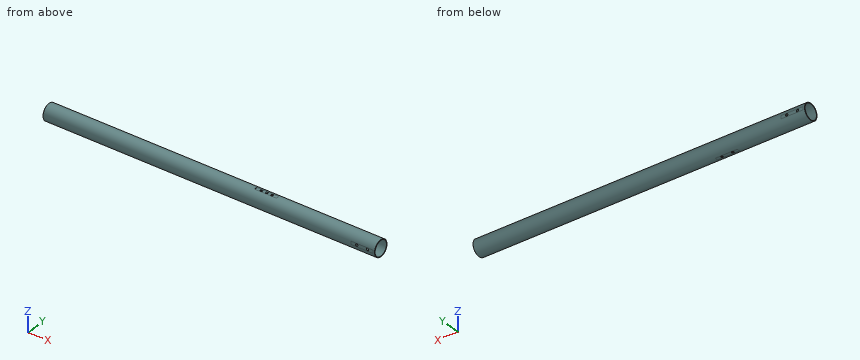
from build123d import *

# Parameters (mm, degrees)
SKETCH1_R                     = 25
SKETCH1_R_2                   = 23
EXTRUDE_THIN1_DEPTH           = 515
EXTRUDE_THIN2_START           = 210
SKETCH1_3_R                   = 25
SKETCH1_3_R_2                 = 21
EXTRUDE_THIN2_DEPTH           = 90
CUT_EXTRUDE1_START            = 24.54
CUT_EXTRUDE1_DEPTH            = 492.672165684
CUT_EXTRUDE2_START            = -24.54
CUT_EXTRUDE2_DEPTH            = 492.672165793
CUT_EXTRUDE3_START            = -24.54
CUT_EXTRUDE3_DEPTH            = 492.672165793
CUT_EXTRUDE4_START            = 24.54
CUT_EXTRUDE4_DEPTH            = 492.672165793
M_0_295_DIAMETER_HOLE3_REACH  = 519.981
M_0_295_DIAMETER_HOLE3_BORE_R = 3.7465
M_0_295_DIAMETER_HOLE4_REACH  = 519.981
M_0_295_DIAMETER_HOLE4_BORE_R = 3.7465
M_0_295_DIAMETER_HOLE5_REACH  = 519.981
M_0_295_DIAMETER_HOLE5_BORE_R = 3.7465
M_0_295_DIAMETER_HOLE6_REACH  = 519.981
M_0_295_DIAMETER_HOLE6_BORE_R = 3.7465
CHAMFER1_SIZE                 = 1


with BuildPart() as part:
    # Sketch1 → Extrude-Thin1 (new, symmetric)
    with BuildSketch(Plane(origin=(0, 0, 0), x_dir=(0, 0, -1), z_dir=(1, 0, 0))):
        Circle(SKETCH1_R)
        Circle(SKETCH1_R_2, mode=Mode.SUBTRACT)
    extrude(amount=EXTRUDE_THIN1_DEPTH, both=True)

    # Sketch1<3> → Extrude-Thin2 (add)
    with BuildSketch(Plane(origin=(0, 0, 0), x_dir=(0, 0, -1), z_dir=(1, 0, 0)).offset(EXTRUDE_THIN2_START)):
        Circle(SKETCH1_3_R)
        Circle(SKETCH1_3_R_2, mode=Mode.SUBTRACT)
    extrude(amount=-EXTRUDE_THIN2_DEPTH)

    # Sketch3 → Cut-Extrude1 (cut, through all)
    with BuildSketch(Plane(origin=(0, 0, 0), x_dir=(1, 0, 0), z_dir=(0, 1, 0)).offset(CUT_EXTRUDE1_START)):
        with BuildLine():
            Line((-491.7775, -17.4725), (-458.1225, -17.4725))
            ThreePointArc((-458.1225, -17.4725), (-440.65, 0), (-458.1225, 17.4725))
            Line((-458.1225, 17.4725), (-491.7775, 17.4725))
            ThreePointArc((-491.7775, 17.4725), (-509.25, 0), (-491.7775, -17.4725))
        make_face()
    extrude(amount=CUT_EXTRUDE1_DEPTH, mode=Mode.SUBTRACT)

    # Sketch8 → Cut-Extrude2 (cut, through all)
    with BuildSketch(Plane.XY.offset(CUT_EXTRUDE2_START)):
        with BuildLine():
            Line((-272.5275, -17.4725), (-238.8725, -17.4725))
            ThreePointArc((-238.8725, -17.4725), (-221.4, 0), (-238.8725, 17.4725))
            Line((-238.8725, 17.4725), (-272.5275, 17.4725))
            ThreePointArc((-272.5275, 17.4725), (-290, 0), (-272.5275, -17.4725))
        make_face()
    extrude(amount=-CUT_EXTRUDE2_DEPTH, mode=Mode.SUBTRACT)

    # Sketch3<3> → Cut-Extrude3 (cut, through all)
    with BuildSketch(Plane(origin=(0, 0, 0), x_dir=(1, 0, 0), z_dir=(0, 1, 0)).offset(CUT_EXTRUDE3_START)):
        with BuildLine():
            ThreePointArc((458.1225, -17.4725), (440.65, 0), (458.1225, 17.4725))
            Line((458.1225, 17.4725), (491.7775, 17.4725))
            ThreePointArc((491.7775, 17.4725), (509.25, 0), (491.7775, -17.4725))
            Line((491.7775, -17.4725), (458.1225, -17.4725))
        make_face()
    extrude(amount=-CUT_EXTRUDE3_DEPTH, mode=Mode.SUBTRACT)

    # Sketch8<4> → Cut-Extrude4 (cut, through all)
    with BuildSketch(Plane.XY.offset(CUT_EXTRUDE4_START)):
        with BuildLine():
            Line((143.8725, -17.4725), (177.5275, -17.4725))
            ThreePointArc((177.5275, -17.4725), (195, 0), (177.5275, 17.4725))
            Line((177.5275, 17.4725), (143.8725, 17.4725))
            ThreePointArc((143.8725, 17.4725), (126.4, 0), (143.8725, -17.4725))
        make_face()
    extrude(amount=CUT_EXTRUDE4_DEPTH, mode=Mode.SUBTRACT)

    # M (0.295) Diameter Hole3 bore → M (0.295) Diameter Hole3 (cut, up to next)
    with BuildSketch(Plane(origin=(0, 24.54, 0), x_dir=(1, 0, 0), z_dir=(0, 1, 0)), mode=Mode.PRIVATE) as m_0_295_diameter_hole3_sk1:
        with Locations((-491.7775, 0)):
            Circle(M_0_295_DIAMETER_HOLE3_BORE_R)
    m_0_295_diameter_hole3_tool1 = extrude(m_0_295_diameter_hole3_sk1.sketch, amount=-M_0_295_DIAMETER_HOLE3_REACH, mode=Mode.PRIVATE) & part.part
    # M (0.295) Diameter Hole3 bore → M (0.295) Diameter Hole3 (cut, up to next)
    with BuildSketch(Plane(origin=(0, 24.54, 0), x_dir=(1, 0, 0), z_dir=(0, 1, 0)), mode=Mode.PRIVATE) as m_0_295_diameter_hole3_sk2:
        with Locations((-458.1225, 0)):
            Circle(M_0_295_DIAMETER_HOLE3_BORE_R)
    m_0_295_diameter_hole3_tool2 = extrude(m_0_295_diameter_hole3_sk2.sketch, amount=-M_0_295_DIAMETER_HOLE3_REACH, mode=Mode.PRIVATE) & part.part
    add(m_0_295_diameter_hole3_tool1.solids().sort_by_distance((-491.7775, 24.54, 0))[0], mode=Mode.SUBTRACT)
    add(m_0_295_diameter_hole3_tool2.solids().sort_by_distance((-458.1225, 24.54, 0))[0], mode=Mode.SUBTRACT)

    # M (0.295) Diameter Hole4 bore → M (0.295) Diameter Hole4 (cut, up to next)
    with BuildSketch(Plane(origin=(0, 0, -24.54), x_dir=(-1, 0, 0), z_dir=(0, 0, -1)), mode=Mode.PRIVATE) as m_0_295_diameter_hole4_sk1:
        with Locations((238.8725, 0)):
            Circle(M_0_295_DIAMETER_HOLE4_BORE_R)
    m_0_295_diameter_hole4_tool1 = extrude(m_0_295_diameter_hole4_sk1.sketch, amount=-M_0_295_DIAMETER_HOLE4_REACH, mode=Mode.PRIVATE) & part.part
    # M (0.295) Diameter Hole4 bore → M (0.295) Diameter Hole4 (cut, up to next)
    with BuildSketch(Plane(origin=(0, 0, -24.54), x_dir=(-1, 0, 0), z_dir=(0, 0, -1)), mode=Mode.PRIVATE) as m_0_295_diameter_hole4_sk2:
        with Locations((272.5275, 0)):
            Circle(M_0_295_DIAMETER_HOLE4_BORE_R)
    m_0_295_diameter_hole4_tool2 = extrude(m_0_295_diameter_hole4_sk2.sketch, amount=-M_0_295_DIAMETER_HOLE4_REACH, mode=Mode.PRIVATE) & part.part
    add(m_0_295_diameter_hole4_tool1.solids().sort_by_distance((-238.8725, 0, -24.54))[0], mode=Mode.SUBTRACT)
    add(m_0_295_diameter_hole4_tool2.solids().sort_by_distance((-272.5275, 0, -24.54))[0], mode=Mode.SUBTRACT)

    # M (0.295) Diameter Hole5 bore → M (0.295) Diameter Hole5 (cut, up to next)
    with BuildSketch(Plane.XY.offset(24.54), mode=Mode.PRIVATE) as m_0_295_diameter_hole5_sk1:
        with Locations((143.8725, 0)):
            Circle(M_0_295_DIAMETER_HOLE5_BORE_R)
    m_0_295_diameter_hole5_tool1 = extrude(m_0_295_diameter_hole5_sk1.sketch, amount=-M_0_295_DIAMETER_HOLE5_REACH, mode=Mode.PRIVATE) & part.part
    # M (0.295) Diameter Hole5 bore → M (0.295) Diameter Hole5 (cut, up to next)
    with BuildSketch(Plane.XY.offset(24.54), mode=Mode.PRIVATE) as m_0_295_diameter_hole5_sk2:
        with Locations((160.7, 0)):
            Circle(M_0_295_DIAMETER_HOLE5_BORE_R)
    m_0_295_diameter_hole5_tool2 = extrude(m_0_295_diameter_hole5_sk2.sketch, amount=-M_0_295_DIAMETER_HOLE5_REACH, mode=Mode.PRIVATE) & part.part
    # M (0.295) Diameter Hole5 bore → M (0.295) Diameter Hole5 (cut, up to next)
    with BuildSketch(Plane.XY.offset(24.54), mode=Mode.PRIVATE) as m_0_295_diameter_hole5_sk3:
        with Locations((177.5275, 0)):
            Circle(M_0_295_DIAMETER_HOLE5_BORE_R)
    m_0_295_diameter_hole5_tool3 = extrude(m_0_295_diameter_hole5_sk3.sketch, amount=-M_0_295_DIAMETER_HOLE5_REACH, mode=Mode.PRIVATE) & part.part
    add(m_0_295_diameter_hole5_tool1.solids().sort_by_distance((143.8725, 0, 24.54))[0], mode=Mode.SUBTRACT)
    add(m_0_295_diameter_hole5_tool2.solids().sort_by_distance((160.7, 0, 24.54))[0], mode=Mode.SUBTRACT)
    add(m_0_295_diameter_hole5_tool3.solids().sort_by_distance((177.5275, 0, 24.54))[0], mode=Mode.SUBTRACT)

    # M (0.295) Diameter Hole6 bore → M (0.295) Diameter Hole6 (cut, up to next)
    with BuildSketch(Plane(origin=(0, -24.54, 0), x_dir=(-1, 0, 0), z_dir=(0, -1, 0)), mode=Mode.PRIVATE) as m_0_295_diameter_hole6_sk1:
        with Locations((-491.7775, 0)):
            Circle(M_0_295_DIAMETER_HOLE6_BORE_R)
    m_0_295_diameter_hole6_tool1 = extrude(m_0_295_diameter_hole6_sk1.sketch, amount=-M_0_295_DIAMETER_HOLE6_REACH, mode=Mode.PRIVATE) & part.part
    # M (0.295) Diameter Hole6 bore → M (0.295) Diameter Hole6 (cut, up to next)
    with BuildSketch(Plane(origin=(0, -24.54, 0), x_dir=(-1, 0, 0), z_dir=(0, -1, 0)), mode=Mode.PRIVATE) as m_0_295_diameter_hole6_sk2:
        with Locations((-458.1225, 0)):
            Circle(M_0_295_DIAMETER_HOLE6_BORE_R)
    m_0_295_diameter_hole6_tool2 = extrude(m_0_295_diameter_hole6_sk2.sketch, amount=-M_0_295_DIAMETER_HOLE6_REACH, mode=Mode.PRIVATE) & part.part
    add(m_0_295_diameter_hole6_tool1.solids().sort_by_distance((491.7775, -24.54, 0))[0], mode=Mode.SUBTRACT)
    add(m_0_295_diameter_hole6_tool2.solids().sort_by_distance((458.1225, -24.54, 0))[0], mode=Mode.SUBTRACT)

    # Chamfer1
    chamfer1_edges = [part.edges().sort_by_distance(p)[0] for p in [
        (-515, 0, 25),
        (-515, 0, 23),
        (515, 0, 25),
        (515, 0, 23),
    ]]
    chamfer(chamfer1_edges, length=CHAMFER1_SIZE - 0.0001)  # a hair under: the kernel refuses the full size


solid = part.part
Read the model definition and answer for the solid it produces. Units are mm, in the model's axes. Round coordinates to 2 decimals unless told otherwise and drop trailing zeros. Write each loop counter-clockwise with the first axis right and the second up, starting at its lowest first coordinate (ties: lowest second). Pieces come first, ordered by that corner, then holes. Notation, with made-up numbers: (-24, -0.75) - (21, -0.75) arc R15 ccw to (21, 6.25) - close; hole circle Ø5 at (18, 62). An arc over 180 degrees is marked (long way). One line per question, with ' | ' between items. Start each with the question number.
1. Each of these flat-tipped pins is pushed along its axis until it touches: pin 1 (3 mm diameter, centred on x = 382.5, z = -15.5, fed in from -Y); pin 2 (10.5 mm diameter, centred on x = -488.5, z = -1.5, fed in from +Y); pin 3 (3 mm diameter, centred on x = -246, y = 1, fed in from -Z); pin 4 (2 mm diameter, centred on y = 5.5, z = 19, fed in from -X). Where does it stop, or does it pass through?
2. Section A-A (x = 326.5) is taken. Determine the outline of the cut face in (y, z), and give its area (3 significant figures).
3. Find the intervals of material crossed by probe 1 along Z at (x, y) = (-329, 4); probe 2 along Z at (x, y) = (-167, 0), in increasing order. Write a range as [from, to].
Filled in:
1) pin 1: y = -20.71 | pin 2: y = 24.54 | pin 3: z = -24.54 | pin 4: through
2) outline: circle Ø50 at (0, 0); hole circle Ø46 at (0, 0) | area: 302 mm²
3) probe 1: [-24.68, -22.65], [22.65, 24.68] | probe 2: [-25, -23], [23, 25]
